The model under review builds one solid part; all positions refer to its coordinate system, in mm. A direction names the side the tool comes from. Round coordinates to 2 decimals unless told otherwise and drop trailing zeros. Order: outer loops, then holes, each group sorted by start corner. A loop starts at its lowest first (then second) coordinate and runs counter-clockwise, first axis right, second up.
1) Clearance check with flat-ended pins moving along their axes: P1, Ø12, axis at x = 35, y = 2.5, coming from the +Z side; P2, Ø3, axis at x = 136.5, z = 4, coming from the +Y side; P3, Ø5, axis at x = 291, y = 0, coming from the +Z side; P4, Ø2, axis at x = 170.5, y = -5.5, coming from the +Z side. State where each tip first meets the part, or that it passes through.
2) Machinability: for faces 1 (the face through (300, -11, 0)), 2 (the face through (300, 11, 0)), 3 (the face through (279, 0, -10)), 4 (the face through (155.652, 10.158, 3.199)), which of the approach directions +Z, -Z, +X, -X, +Y, -Y give a long, thin tool a straight path to every point of the face, cutting with its end or side? Answer none if there is none.
3) To check wall thickness, follow L1, parallel to Z at x = 37.5, y = 0; L2, parallel to Z at x = 68.5, y = -0.5; L3, parallel to X at y = 8, z = 8.25. State the ranges of each line that lie inside material, in increasing order.
4) Mouldability with a two-part tool opening along Y and no side actions: class faces 5 (the face through (24, 13.5, -3)), 6 (the face through (26, -4, 0)), 7 (the face through (154.24, -2.17, -9.76)), 8 (the face through (8.57, -2.38, -10.74)) as pulls with the +Y half, pulls with the -Y half, needs draft (parallel to the pull), parting line crosses it, or undercut.
5) Consider section A-A (x = 63). Give the boundary of the cut face in (y, z).
Autodesk Inventor part; units mm, degrees
ref_plane "FDT_FRONT_XY" through (20, 0, 0) normal (1, 0, 0) x (0, 0, -1)
ref_plane "FDT_FRONT_YZ" through (20, 0, 0) normal (0, 0, -1) x (0, 1, 0)
ref_plane "FDT_FRONT_ZX" through (20, 0, 0) normal (0, 1, 0) x (1, 0, 0)
sketch "Sketch_1" plane through (0, 0, 0) normal (0, 0, 1) x (1, 0, 0)
  line L0 (20, 0) -> (0, 0)
  line L1 (0, 0) -> (0, 9.8)
  line L2 (0, 9.8) -> (0.2, 10)
  line L3 (0.2, 10) -> (1, 10)
  line L4 (1, 10) -> (2, 11)
  line L5 (2, 11) -> (14.95, 11)
  line L6 (14.95, 11) -> (15.8657, 10.0843)
  arc A0 (15.8657, 10.0843) -> (16.4314, 9.85) centre (16.4314, 10.65) ccw
  line L7 (16.4314, 9.85) -> (17.2, 9.85)
  arc A1 (17.2, 9.85) -> (18, 10.65) centre (17.2, 10.65) ccw
  line L8 (18, 10.65) -> (18, 11)
  line L9 (18, 11) -> (20, 11)
  line L10 (20, 11) -> (20, 0)
  line L11 (20, 0) -> (0, 0)
revolve "Revolution1" add sketch "Sketch_1" angle 360 about axis through (20, 0, 0) along (1, 0, 0)
thread "Thread1"
sketch "Sketch_2" plane through (20, 0, 0) normal (1, 0, 0) x (0, 0, -1)
  arc A0 (-7.3859, 11.3004) -> (7.3859, 11.3004) centre (0, 0) ccw
  arc A1 (7.25, 11.5515) -> (7.3859, 11.3004) centre (7.55, 11.5515) ccw
  line L0 (7.25, 11.5515) -> (7.25, 13.1)
  arc A2 (7.25, 13.1) -> (6.85, 13.5) centre (6.85, 13.1) ccw
  line L1 (6.85, 13.5) -> (-6.85, 13.5)
  arc A3 (-6.85, 13.5) -> (-7.25, 13.1) centre (-6.85, 13.1) ccw
  line L2 (-7.25, 13.1) -> (-7.25, 11.5515)
  arc A4 (-7.3859, 11.3004) -> (-7.25, 11.5515) centre (-7.55, 11.5515) ccw
extrude "Extrusion1" add sketch "Sketch_2" along normal blind 16
sketch "Sketch_3" plane through (0, 0, 0) normal (0, 0, 1) x (1, 0, 0)
  line L0 (272, 0) -> (36, 0)
  line L1 (36, 0) -> (36, 10.65)
  line L2 (36, 10.65) -> (272, 10.65)
  line L3 (272, 10.65) -> (272, 0)
  line L4 (272, 0) -> (36, 0)
revolve "Revolution2" add sketch "Sketch_3" angle 360 about axis through (272, 0, 0) along (1, 0, 0)
sketch "Sketch_16" plane through (272, 0, 0) normal (1, 0, 0) x (0, 0, -1)
  arc A0 (-7.3859, 11.3004) -> (7.3859, 11.3004) centre (0, 0) ccw
  arc A1 (7.25, 11.5515) -> (7.3859, 11.3004) centre (7.55, 11.5515) ccw
  line L0 (7.25, 11.5515) -> (7.25, 13.1)
  arc A2 (7.25, 13.1) -> (6.85, 13.5) centre (6.85, 13.1) ccw
  line L1 (6.85, 13.5) -> (-6.85, 13.5)
  arc A3 (-6.85, 13.5) -> (-7.25, 13.1) centre (-6.85, 13.1) ccw
  line L2 (-7.25, 13.1) -> (-7.25, 11.5515)
  arc A4 (-7.3859, 11.3004) -> (-7.25, 11.5515) centre (-7.55, 11.5515) ccw
extrude "Extrusion2" add sketch "Sketch_16" along normal blind 16
sketch "Sketch_23" plane through (0, 0, 0) normal (0, 0, 1) x (1, 0, 0)
  line L0 (308, 0) -> (288, 0)
  line L1 (288, 0) -> (288, 11)
  line L2 (288, 11) -> (290, 11)
  line L3 (290, 11) -> (290, 10.65)
  arc A0 (290, 10.65) -> (290.8, 9.85) centre (290.8, 10.65) ccw
  line L4 (290.8, 9.85) -> (291.5686, 9.85)
  arc A1 (291.5686, 9.85) -> (292.1343, 10.0843) centre (291.5686, 10.65) ccw
  line L5 (292.1343, 10.0843) -> (293.05, 11)
  line L6 (293.05, 11) -> (306, 11)
  line L7 (306, 11) -> (307, 10)
  line L8 (307, 10) -> (307.8, 10)
  line L9 (307.8, 10) -> (308, 9.8)
  line L10 (308, 9.8) -> (308, 0)
  line L11 (308, 0) -> (288, 0)
revolve "Revolution3" add sketch "Sketch_23" angle 360 about axis through (308, 0, 0) along (1, 0, 0)
thread "Thread2"
sketch "Sketch_6" plane through (0, 0, 0) normal (0, 1, 0) x (-1, 0, 0)
  line L0 (-279, -24) -> (-279, -8)
  line L1 (-279, -8) -> (-308, -8)
  line L2 (-308, -8) -> (-308, 8)
  line L3 (-308, 8) -> (-279, 8)
  line L4 (-279, 8) -> (-279, 24)
  line L5 (-279, 24) -> (-324, 24)
  line L6 (-324, 24) -> (-324, -24)
  line L7 (-324, -24) -> (-279, -24)
extrude "Extrusion3" cut sketch "Sketch_6" along normal mid plane 27
sketch "Sketch7" plane through (306, -7.5498, -8) normal (0, 0, -1) x (-1, 0, 0)
  point P0 (15, 7.5498)
hole "Hole1" at (291, 0, -8) direction (0, 0, 1) diameter 8 depth 16
sketch "Sketch8" plane through (20, 13.5, 6.85) normal (0, 1, 0) x (1, 0, 0)
  point P0 (8.2, 6.85)
hole "Hole2" at (28.2, 13.5, 0) direction (0, -1, 0) diameter 8.566 depth 13.5 countersink diameter 9.728 countersink angle 90
sketch "Sketch9" plane through (272, 13.5, 6.85) normal (0, 1, 0) x (1, 0, 0)
  point P0 (7.8, 6.85)
hole "Hole3" at (279.8, 13.5, 0) direction (0, -1, 0) diameter 8.566 depth 16 tip angle 120 countersink diameter 9.728 countersink angle 90
sketch "Sketch_64" plane through (0, 0, 0) normal (0, 0, 1) x (1, 0, 0)
  line L0 (255.3, 0) -> (-4, 0)
  line L1 (-4, 0) -> (-4, 4)
  line L2 (-4, 4) -> (50.3, 4)
  line L3 (50.3, 4) -> (50.3, 10)
  line L4 (50.3, 10) -> (255.3, 10)
  line L5 (255.3, 10) -> (255.3, 0)
  line L6 (255.3, 0) -> (-4, 0)
revolve "Revolution4" cut sketch "Sketch_64" angle 360 about axis through (255.3, 0, 0) along (1, 0, 0)
ref_plane "FDT_FRONT_XY" through (20, 0, 0) normal (1, 0, 0) x (0, 0, -1)
ref_plane "FDT_FRONT_YZ" through (20, 0, 0) normal (0, 0, -1) x (0, 1, 0)
ref_plane "FDT_FRONT_ZX" through (20, 0, 0) normal (0, 1, 0) x (1, 0, 0)
ref_plane "FDT_QSFRONT_XY" through (28.2, 13.5, 0) normal (0, 1, 0) x (0, 0, 1)
ref_plane "FDT_QSFRONT_YZ" through (28.2, 13.5, 0) normal (0, 0, 1) x (1, 0, 0)
ref_plane "FDT_QSFRONT_ZX" through (28.2, 13.5, 0) normal (1, 0, 0) x (0, 1, 0)
ref_plane "FDT_QSREAR_XY" through (279.8, 13.5, 0) normal (0, 1, 0) x (0, 0, 1)
ref_plane "FDT_QSREAR_YZ" through (279.8, 13.5, 0) normal (0, 0, 1) x (1, 0, 0)
ref_plane "FDT_QSREAR_ZX" through (279.8, 13.5, 0) normal (1, 0, 0) x (0, 1, 0)
ref_plane "FDT_REAR_XY" through (288, 0, 0) normal (-1, 0, 0) x (0, 0, -1)
ref_plane "FDT_REAR_YZ" through (288, 0, 0) normal (0, 0, -1) x (0, -1, 0)
ref_plane "FDT_REAR_ZX" through (288, 0, 0) normal (0, -1, 0) x (-1, 0, 0)
ref_plane "FDT_SMBR1_XY" through (45.5, 0, 0) normal (-1, 0, 0) x (0, 0, 1)
ref_plane "FDT_SMBR1_YZ" through (45.5, 0, 0) normal (0, 0, 1) x (0, 1, 0)
ref_plane "FDT_SMBR1_ZX" through (45.5, 0, 0) normal (0, 1, 0) x (-1, 0, 0)
ref_plane "FDT_SMBR2_XY" through (262.5, 0, 0) normal (-1, 0, 0) x (0, 0, 1)
ref_plane "FDT_SMBR2_YZ" through (262.5, 0, 0) normal (0, 0, 1) x (0, 1, 0)
ref_plane "FDT_SMBR2_ZX" through (262.5, 0, 0) normal (0, 1, 0) x (-1, 0, 0)
ref_plane "FDT_SWIVELAXIS_XY" through (291, 0, 0) normal (0, 0, 1) x (1, 0, 0)
ref_plane "FDT_SWIVELAXIS_YZ" through (291, 0, 0) normal (1, 0, 0) x (0, 1, 0)
ref_plane "FDT_SWIVELAXIS_ZX" through (291, 0, 0) normal (0, 1, 0) x (0, 0, 1)
ref_plane "NUT_XY" through (6.5, 0, 0) normal (1, 0, 0) x (0, 0, -1)
ref_plane "NUT_YZ" through (6.5, 0, 0) normal (0, 0, -1) x (0, 1, 0)
ref_plane "NUT_ZX" through (6.5, 0, 0) normal (0, 1, 0) x (1, 0, 0)
ref_plane "ZR_XY" through (0, 0, 0) normal (1, 0, 0) x (0, 0, -1)
ref_plane "ZR_YZ" through (0, 0, 0) normal (0, 0, -1) x (0, 1, 0)
ref_plane "ZR_ZX" through (0, 0, 0) normal (0, 1, 0) x (1, 0, 0)
ref_plane "ZYL_XY" through (20, 0, 0) normal (1, 0, 0) x (0, 0, -1)
ref_plane "ZYL_YZ" through (20, 0, 0) normal (0, 0, -1) x (0, 1, 0)
ref_plane "ZYL_ZX" through (20, 0, 0) normal (0, 1, 0) x (1, 0, 0)
properties part number "559278 DSNU-20-200-PPS---(A----0-ZR)"
Answer below:
1. P1: stops at z = 13.5
1. P2: stops at y = 10.35
1. P3: passes through
1. P4: stops at z = 9.65
2. face 1: +X, -Y
2. face 2: +X, +Y
2. face 3: -Z, +X, +Y, -Y
2. face 4: none
3. L1: z = -10.65 to -4, 4 to 10.65
3. L2: z = -10.64 to -9.99, 9.99 to 10.64
3. L3: x = 20 to 36, 272 to 279
4. face 5: pulls with the +Y half
4. face 6: undercut
4. face 7: undercut
4. face 8: parting line crosses it
5. outline: circle Ø21.3 at (0, 0); hole circle Ø20 at (0, 0)
